Could you check a few things on this model? Use its own coordinates, in mm. Give positions to 0.01 mm unless a question says otherwise; leave off trailing zeros. Loops run counter-clockwise (first coordinate to the right, second up) from the corner with the lowest first, then second, coordinate; pieces in that order, holes last. Notation, with made-up numbers: (87, 47.25) - (113, 47.25) arc R9 cw to (113, 61.25) - close; hole circle Ø5 at (-4, 5). An arc over 180 degrees is marked (long way). Answer in a Markdown table with one row per item. Add a question column.
Autodesk Inventor part; units mm, degrees
ref_plane "YZ Plane" through (0, 0, 0) normal (1, 0, 0) x (0, 1, 0)
ref_plane "XZ Plane" through (0, 0, 0) normal (0, 1, 0) x (-1, 0, 0)
ref_plane "XY Plane" through (0, 0, 0) normal (0, 0, 1) x (1, 0, 0)
sketch "Sketch1" plane through (0, 0, 0) normal (0, 0, 1) x (1, 0, 0)
  circle A0 centre (0, 0) radius 1.8
  line L0 (-3.5, 3.5) -> (3.5, 3.5)
  line L1 (3.5, 3.5) -> (3.5, -3.5)
  line L2 (3.5, -3.5) -> (-3.5, -3.5)
  line L3 (-3.5, -3.5) -> (-3.5, 3.5)
  point P0 (3.5, 0)
  point P1 (0, 3.5)
  dimension "d0" = 3.6
  dimension "d24" = 7
extrude "Extrusion1" add sketch "Sketch1" along normal blind 13.5
fillet "Fillet3" radius 2 4 edges at (3.5, 3.5, 6.75) (3.5, -3.5, 6.75) (-3.5, -3.5, 6.75) (-3.5, 3.5, 6.75)
chamfer "Chamfer4" distance 0.4 angle 45 18 edges at (-2.9142, -2.9142, 13.5) (-3.5, 0, 13.5) (-2.9142, 2.9142, 13.5) (0, 3.5, 13.5) (2.9142, 2.9142, 13.5) (3.5, 0, 13.5) (2.9142, -2.9142, 13.5) (0, -3.5, 13.5) (2.9142, -2.9142, 0) (3.5, 0, 0) (2.9142, 2.9142, 0) (0, 3.5, 0) (-2.9142, 2.9142, 0) (-3.5, 0, 0) (-2.9142, -2.9142, 0) (0, -3.5, 0) (-1.8, 0, 13.5) (-1.8, 0, 0)
properties part number "shaft-15mm-squareipt" material "ABS Plastic"
(1) We'd pull the mould along X, two halves only. Please class faces 1 (the cylindrical face through (1.717, -0.541, 6.661)), 2 (the conical face through (2.699, -2.725, 0.114)), 3 (the conical face through (-2.699, 2.725, 0.114)): pulls with the +X half, pulls with the -X half, needs draft (parallel to the pull), parting line crosses it, or undercut.
(2) I want a section at B-B on z = 10.25. Please give me the cut outline in (x, y), then the cut area to 3 significant figures.
(3) Please list where these lines run through material, in increasing order: line 1 (Y direction, x = 0, z = 7); line 2 (X direction, y = 0.5, z = 2.25); line 3 (X direction, y = -0.25, z = 5).
(4) I want a section at A-A on x = 0. Please give me the cut outline in (y, z).
Reported:
| question | item | result |
|---|---|---|
| 1 | face 1 | undercut |
| 1 | face 2 | pulls with the +X half |
| 1 | face 3 | pulls with the -X half |
| 2 | outline | (-3.5, -1.5) arc R2 ccw to (-1.5, -3.5) - (1.5, -3.5) arc R2 ccw to (3.5, -1.5) - (3.5, 1.5) arc R2 ccw to (1.5, 3.5) - (-1.5, 3.5) arc R2 ccw to (-3.5, 1.5) - close; hole circle Ø3.6 at (0, 0) |
| 2 | area | 35.4 mm² |
| 3 | line 1 | -3.5 to -1.8, 1.8 to 3.5 |
| 3 | line 2 | -3.5 to -1.73, 1.73 to 3.5 |
| 3 | line 3 | -3.5 to -1.78, 1.78 to 3.5 |
| 4 | outline | (-3.5, 0.4) - (-3.1, 0) - (-2.2, 0) - (-1.8, 0.4) - (-1.8, 13.1) - (-2.2, 13.5) - (-3.1, 13.5) - (-3.5, 13.1) - close; (1.8, 0.4) - (2.2, 0) - (3.1, 0) - (3.5, 0.4) - (3.5, 13.1) - (3.1, 13.5) - (2.2, 13.5) - (1.8, 13.1) - close |
